from build123d import *

# Parameters (mm, degrees)
F0_R      = 1.5
F1_DEPTH  = 5
F3_W      = 2
F3_H      = 8
F4_DEPTH  = 45
F6_W      = 20
F6_H      = 6.2
F7_DEPTH  = 25
F9_W      = 4
F9_H      = 8
F10_DEPTH = 40


with BuildPart() as f1:
    # F0 (on Front) → F1 (new body, symmetric)
    with BuildSketch(Plane.XZ):
        with BuildLine():
            ThreePointArc((30, -4), (34, 0), (30, 4))
            Line((30, 4), (-30, 4))
            ThreePointArc((-30, 4), (-34, 0), (-30, -4))
            Line((-30, -4), (30, -4))
        make_face()
        with Locations((-30, 0)):
            Circle(F0_R, mode=Mode.SUBTRACT)
        Circle(F0_R, mode=Mode.SUBTRACT)
        with Locations((30, 0)):
            Circle(F0_R, mode=Mode.SUBTRACT)
    extrude(amount=F1_DEPTH, both=True)

    # F3 (on offset) → F4 (cut)
    with BuildSketch(Plane.YZ.offset(64)):
        Rectangle(F3_W, F3_H)
    extrude(amount=-F4_DEPTH, mode=Mode.SUBTRACT)

    # F6 (on face) → F7 (cut)
    with BuildSketch(Plane.XY.offset(4)):
        Rectangle(F6_W, F6_H)
    extrude(amount=-F7_DEPTH, mode=Mode.SUBTRACT)

    # F9 (on offset) → F10 (cut)
    with BuildSketch(Plane.YZ.offset(-64)):
        Rectangle(F9_W, F9_H)
    extrude(amount=F10_DEPTH, mode=Mode.SUBTRACT)


solid = f1.part
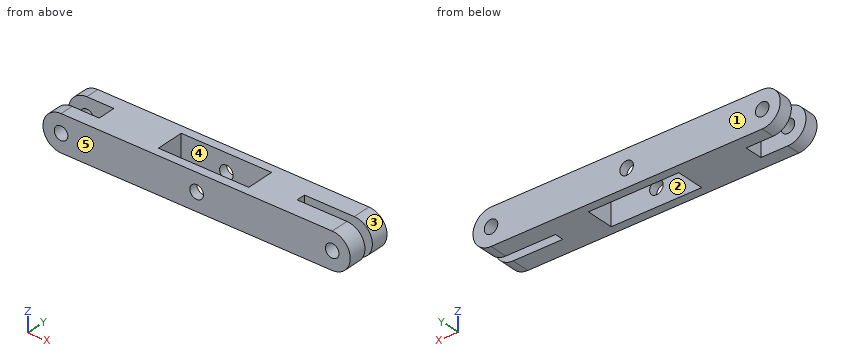
Model file for the job. Use its own axes, mm. Face numbers are marked on the shaded views. A direction names the side the tool comes from. Give positions to 0.01 mm unless a question says otherwise; leave off trailing zeros. Order: outer loops, then holes, each group sorted by start corner. A loop starts at its lowest first (then second) coordinate and runs counter-clockwise, first axis right, second up. Notation, with made-up numbers: M 54,-25.75 L 86,-25.75 A14 cw 86,-15.75 Z; hole C 32.5,74 d4. An arc over 180 degrees is marked long. Put each result on its own line as item: value. Start each with the question number.
(1) Pin check, flat tips, straight feed: pin 1 Ø2.5 at (x, z) = (-30, 0) entering from -Y; pin 2 Ø1.5 at (y, z) = (-1.5, 1) entering from -X; pin 3 Ø1 at (y, z) = (-2, -3) entering from -X. Stop position of each tip, or through.
(2) Band-saw the part on C-C on x = 0. Give the cut face in (y, z).
(3) Band-saw the part on A-A on x = -7. Give the cut face in (y, z), then the cut area to 3 significant figures.
(4) Band-saw the part on B-B on y = 3.75. Give the cut face in (x, z), then the cut area to 3 significant figures.
(5) Drill centre lines: L1, parallel to X at y = -4.35, z = 0; L2, parallel to Y at x = 24.5, z = -3.25; L3, parallel to Z at x = 30, y = -4. Where is each one in solid material? Low to high. Write a range as [from, to].
(6) Pull direction X, two halves, no side cores. Call the marked faces 3, 4 and 5: released by +X, released by -X, zero draft, split by the parting line, or undercut.
(7) Tool access for the marked faces 1 and 2: list every direction of +Z, -Z, +X, -X, +Y, -Y with a clear straight run to the whole face (end or side of a thin tool).
(8) Band-saw the part on D-D on y = 0. Give the cut face in (x, z).
Results below:
1. pin 1: passes through
1. pin 2: stops at x = -33.98
1. pin 3: stops at x = -33.12
2. outline: M -5,-4 L -3.1,-4 L -3.1,-1.5 L -5,-1.5 Z; M -5,1.5 L -3.1,1.5 L -3.1,4 L -5,4 Z; M 3.1,-4 L 5,-4 L 5,-1.5 L 3.1,-1.5 Z; M 3.1,1.5 L 5,1.5 L 5,4 L 3.1,4 Z
3. outline: M -5,-4 L -3.1,-4 L -3.1,4 L -5,4 Z; M 3.1,-4 L 5,-4 L 5,4 L 3.1,4 Z
3. area: 30.4 mm2
4. outline: M -30,-4 L 30,-4 A4 ccw 30,4 L -30,4 A4 ccw Z; hole C -30,0 d3; hole C 0,0 d3; hole C 30,0 d3
4. area: 509 mm2
5. L1: x = [-34, -31.5], [-28.5, -1.5], [1.5, 28.5], [31.5, 34]
5. L2: y = [-5, -1], [1, 5]
5. L3: z = [-4, -1.5], [1.5, 4]
6. face 3: released by +X
6. face 4: undercut
6. face 5: zero draft
7. face 1: +Z, -Z, +X, -X, +Y
7. face 2: +Z, -Z
8. outline: M -24,-4 L -10,-4 L -10,4 L -24,4 Z; M 10,-4 L 19,-4 L 19,4 L 10,4 Z
